Geometry check sheet. Reference: the model listing, model coordinates, mm. A direction names the side the tool comes from. Coordinates: 2 decimals unless noted, no trailing zeros. Write each loop counter-clockwise with the first axis right and the second up, starting at its lowest first coordinate (ties: lowest second). Pieces come first, ordered by that corner, then holes. Notation, with made-up numbers: M 88.25,-6.75 L 134.25,-6.75 A17 cw 134.25,13.25 Z; hole C 47.25,46 d2. An arc over 180 degrees is marked long. Write each question's results on one line, items separated by ' | '.
```python
from build123d import *

# Parameters (mm, degrees)
F0_W     = 57.15
F0_H     = 25.4
F1_DEPTH = 12.7
F2_W     = 63.5
F2_H     = 31.75
F2_W_2   = 57.15
F2_H_2   = 25.4
F3_DEPTH = 6.35
F4_R     = 7.9375
F5_DEPTH = 19.051
F6_W     = 52.07
F6_H     = 20.32
F6_R     = 7.9375
F7_DEPTH = 12.7


with BuildPart() as f1:
    # F0 (on Top) → F1 (new body)
    with BuildSketch(Plane.XY):
        Rectangle(F0_W, F0_H)
    extrude(amount=F1_DEPTH)

    # F2 (on face) → F3 (join)
    with BuildSketch(Plane.XY.offset(12.7)):
        Rectangle(F2_W, F2_H)
        Rectangle(F2_W_2, F2_H_2, mode=Mode.SUBTRACT)
        Rectangle(F2_W_2, F2_H_2)
    extrude(amount=F3_DEPTH)

    # F4 (on face) → F5 (cut, through all)
    with BuildSketch(Plane.XY.offset(19.05)):
        with Locations((-15.875, 0)):
            Circle(F4_R)
        with Locations((15.875, 0)):
            Circle(F4_R)
    extrude(amount=-F5_DEPTH, mode=Mode.SUBTRACT)

    # F6 (on face) → F7 (cut)
    with BuildSketch(Plane(origin=(0, 0, 0), x_dir=(1, 0, 0), z_dir=(0, 0, -1))):
        Rectangle(F6_W, F6_H)
        with Locations((-15.875, 0)):
            Circle(F6_R, mode=Mode.SUBTRACT)
        with Locations((15.875, 0)):
            Circle(F6_R, mode=Mode.SUBTRACT)
        with Locations((15.875, 0)):
            Circle(F6_R)
    extrude(amount=-F7_DEPTH, mode=Mode.SUBTRACT)


solid = f1.part
```
Q1. Sectioned sample at B-B on x = -27. Record the cut outline in (y, z) (3 decimals), and give its area (3 significant figures).
Geometry check:
outline: M -15.875,12.7 L -12.7,12.7 L -12.7,0 L 12.7,0 L 12.7,12.7 L 15.875,12.7 L 15.875,19.05 L -15.875,19.05 Z | area: 524 mm2
Q2. Depth check by flat-ended pin: P1, Ø9.5, axis at x = 13, y = -1.5, coming from the -Z side; P2, Ø1.5, axis at y = 8, z = 3.5, coming from the -X side (3 decimals); P3, Ø6.5, axis at x = 10, z = 7.5, coming from the +Y side. Enter the tip coordinate at first touch or a pass-through.
Geometry check:
P1: stops at z = 12.7 | P2: stops at x = -28.575 | P3: stops at y = 12.7
Q3. Sectioned sample at D-D on x = 9.5. Record the cut outline in (y, z) (3 decimals).
Geometry check:
outline: M -15.875,12.7 L -12.7,12.7 L -12.7,0 L -10.16,0 L -10.16,12.7 L -4.729,12.7 L -4.729,19.05 L -15.875,19.05 Z; M 4.729,12.7 L 10.16,12.7 L 10.16,0 L 12.7,0 L 12.7,12.7 L 15.875,12.7 L 15.875,19.05 L 4.729,19.05 Z
Q4. Mould release check, pull along X, two halves, no side actions. Record for faces 1 (the flat face through (-3, -13, 12.7)), 2 (the flat face through (26.035, 0, 6)), 3 (the flat face through (-31.75, 0, 16)): pulls with the +X half, pulls with the -X half, needs draft (parallel to the pull), parting line crosses it, or undercut.
Geometry check:
face 1: needs draft | face 2: undercut | face 3: pulls with the -X half
Q5. Scan lines: probe 1 along Y at (x, z) = (-23.5, 8); probe 2 along X at (y, z) = (-6, 8.25) (3 decimals); probe 3 along Z at (x, y) = (1, 1.5). Record each from-to range of solid material in increasing order.
Geometry check:
probe 1: y = -12.7 to -10.16, 10.16 to 12.7 | probe 2: x = -28.575 to -26.035, 26.035 to 28.575 | probe 3: z = 12.7 to 19.05
Q6. Sectioned sample at A-A on y = 0. Give the number of separate pieces and of enclosed holes in the cut face, and give its area (3 significant figures).
Geometry check:
separate pieces: 3 | enclosed holes: 0 | area: 266 mm2
Q7. Access from +Z, -Z, +X, -X, +Y, -Y to the whole of each face (thin tool, end or side, straight path). Record for faces 4 (the flat face through (0, -12.7, 6)), 5 (the flat face through (0, 10.16, 6)), 6 (the flat face through (28.575, 0, 6)), 7 (the flat face through (0, 12.7, 6)), 8 (the flat face through (-28.575, 0, 6)).
Geometry check:
face 4: -Z, +X, -X, -Y | face 5: -Z | face 6: -Z, +X, +Y, -Y | face 7: -Z, +X, -X, +Y | face 8: -Z, -X, +Y, -Y
